```python
from build123d import *

# Parameters (mm, degrees)
SKETCH1_R           = 3.175
BOSS_EXTRUDE1_DEPTH = 3.175
FILLET1_R           = 12.7


with BuildPart() as part:
    # Sketch1 → Boss-Extrude1 (new body)
    with BuildSketch(Plane.XY):
        Polygon((0, 0), (0, 101.6), (25.4, 101.6), (25.4, 76.2), (76.2, 76.2), (76.2, 25.4), (25.4, 25.4), (25.4, 0), align=None)
        with Locations((12.7, 88.9)):
            Circle(SKETCH1_R, mode=Mode.SUBTRACT)
        with Locations((12.7, 63.5)):
            Circle(SKETCH1_R, mode=Mode.SUBTRACT)
        with Locations((12.7, 38.1)):
            Circle(SKETCH1_R, mode=Mode.SUBTRACT)
        with Locations((12.7, 12.7)):
            Circle(SKETCH1_R, mode=Mode.SUBTRACT)
        with Locations((38.1, 63.5)):
            Circle(SKETCH1_R, mode=Mode.SUBTRACT)
        with Locations((38.1, 38.1)):
            Circle(SKETCH1_R, mode=Mode.SUBTRACT)
        with Locations((63.5, 63.5)):
            Circle(SKETCH1_R, mode=Mode.SUBTRACT)
        with Locations((63.5, 38.1)):
            Circle(SKETCH1_R, mode=Mode.SUBTRACT)
    extrude(amount=BOSS_EXTRUDE1_DEPTH)

    # Fillet1
    fillet1_edges = [part.edges().sort_by_distance(p)[0] for p in [
        (25.4, 76.2, 1.5875),
        (25.4, 25.4, 1.5875),
    ]]
    fillet(fillet1_edges, radius=FILLET1_R)


solid = part.part
```
Part model, mm, in its own coordinate system. A direction names the side the tool comes from. Give positions to 0.01 mm unless a question says otherwise; leave off trailing zeros. Order: outer loops, then holes, each group sorted by start corner. A loop starts at its lowest first (then second) coordinate and runs counter-clockwise, first axis right, second up. Notation, with made-up numbers: (61, -17) - (75, -17) arc R28 cw to (75, 16) - close; hole circle Ø6 at (-22.5, -16.75). An arc over 180 degrees is marked (long way). Use one line per item in the form item = value.
Item 1: Slice it at D-D on z = 2.15. Count the separate pieces of the cut face and the enclosed holes in it, and give its area (3 significant figures).
Solution:
separate_pieces = 1
enclosed_holes = 8
area = 4,980 mm2
Item 2: Probe probe 1 along Y at (x, z) = (12.7, 1.2) (3 decimals); probe 2 along Y at (x, z) = (35.5, 1.85); probe 3 along X at (y, z) = (62, 0.75). List the from-to ranges inside material, lowest first. Write a range as from..to.
Solution:
probe_1 = 0..9.525, 15.875..34.925, 41.275..60.325, 66.675..85.725, 92.075..101.6
probe_2 = 25.13..36.28, 39.92..61.68, 65.32..76.47
probe_3 = 0..9.9, 15.5..35.3, 40.9..60.7, 66.3..76.2
Item 3: Slice it at C-C on x = 12.7. Give the cut face in (y, z) (3 decimals), and give its area (3 significant figures).
Solution:
outline = (0, 0) - (9.525, 0) - (9.525, 3.175) - (0, 3.175) - close; (15.875, 0) - (34.925, 0) - (34.925, 3.175) - (15.875, 3.175) - close; (41.275, 0) - (60.325, 0) - (60.325, 3.175) - (41.275, 3.175) - close; (66.675, 0) - (85.725, 0) - (85.725, 3.175) - (66.675, 3.175) - close; (92.075, 0) - (101.6, 0) - (101.6, 3.175) - (92.075, 3.175) - close
area = 242 mm2
Item 4: Slice it at A-A on x = 63.5. Give the cut face in (y, z) (3 decimals).
Solution:
outline = (25.4, 0) - (34.925, 0) - (34.925, 3.175) - (25.4, 3.175) - close; (41.275, 0) - (60.325, 0) - (60.325, 3.175) - (41.275, 3.175) - close; (66.675, 0) - (76.2, 0) - (76.2, 3.175) - (66.675, 3.175) - close
Item 5: Slice it at B-B on y = 38.1. Give the cut face in (x, z) (3 decimals).
Solution:
outline = (0, 0) - (9.525, 0) - (9.525, 3.175) - (0, 3.175) - close; (15.875, 0) - (34.925, 0) - (34.925, 3.175) - (15.875, 3.175) - close; (41.275, 0) - (60.325, 0) - (60.325, 3.175) - (41.275, 3.175) - close; (66.675, 0) - (76.2, 0) - (76.2, 3.175) - (66.675, 3.175) - close
Item 6: Pin check, flat tips, straight feed: pin 1 Ø4 at (x, y) = (38.1, 63.5) entering from -Z; pin 2 Ø10 at (x, y) = (12.7, 38.1) entering from +Z (3 decimals); pin 3 Ø1.6 at (x, z) = (53, 2.5) entering from +Y. Stop position of each tip, or through.
Solution:
pin_1 = through
pin_2 = 3.175
pin_3 = 76.2
Item 7: Two-plate mould, pull along X, no slides. Class faces 1 (the face through (25.4, 6, 2)), 2 (the face through (10.36, 65.646, 1.565)), 3 (the face through (0, 50, 2)), 4 (the face through (57, 76.2, 2)): released by +X, released by -X, zero draft, split by the parting line, or undercut.
Solution:
face_1 = released by +X
face_2 = undercut
face_3 = released by -X
face_4 = zero draft
Item 8: Which spindle directions (+Z, -Z, +X, -X, +Y, -Y) get a long thin tool onto all of the face, cutting with end or side? Do faces 5 (the face through (25.4, 95, 2)), 6 (the face through (10.18, 10.77, 1.57)). Say none if no direction does.
Solution:
face_5 = +Z, -Z, +X, +Y
face_6 = +Z, -Z
